Part model, mm, in its own coordinate system. A direction names the side the tool comes from. Round coordinates to 2 decimals unless told otherwise and drop trailing zeros. Order: outer loops, then holes, each group sorted by start corner. A loop starts at its lowest first (then second) coordinate and runs counter-clockwise, first axis right, second up. Notation, with made-up numbers: (1.25, -31) -> (51.25, -31) arc R24 ccw to (51.25, -12) -> close; hole circle Ø10 at (17, 19.25). An arc over 180 degrees is marked (long way). Answer as a JSON object with one key per item and string values. Group by question number.
```python
from build123d import *

# Parameters (mm, degrees)
SKETCH2_R           = 7.5
BOSS_EXTRUDE2_DEPTH = 80
SKETCH5_W           = 16
SKETCH5_H           = 60
CUT_EXTRUDE5_DEPTH  = 5
CUT_EXTRUDE6_DEPTH  = 28
CUT_EXTRUDE7_DEPTH  = 28
SKETCH8_R           = 2
CUT_EXTRUDE8_DEPTH  = 5


with BuildPart() as part:
    # Sketch2 → Boss-Extrude2 (new body)
    with BuildSketch(Plane.XY):
        Polygon((8, 0), (15, 0), (23.160384018, -17.5), (40, -17.5), (40, 17.5), (0, 17.5), (-40, 17.5), (-40, -17.5), (-23.160384018, -17.5), (-15, 0), (-8, 0), (-8, -5), (8, -5), align=None)
        with Locations((-27.5, 0)):
            Circle(SKETCH2_R, mode=Mode.SUBTRACT)
        with Locations((27.5, 0)):
            Circle(SKETCH2_R, mode=Mode.SUBTRACT)
        Polygon((-3, 0), (-3, -2.5), (3, -2.5), (3, 0), (3, 2.5), (-3, 2.5), align=None, mode=Mode.SUBTRACT)
    extrude(amount=-BOSS_EXTRUDE2_DEPTH)

    # Sketch5 → Cut-Extrude5 (cut)
    with BuildSketch(Plane(origin=(0, -5, 0), x_dir=(-1, 0, 0), z_dir=(0, -1, 0))):
        with Locations((0, 40)):
            Rectangle(SKETCH5_W, SKETCH5_H)
    extrude(amount=-CUT_EXTRUDE5_DEPTH, mode=Mode.SUBTRACT)

    # Sketch6 → Cut-Extrude6 (cut)
    with BuildSketch(Plane.XY):
        Polygon((-40, 12.5), (-40, -17.5), (-23.160384018, -17.5), (-15, 0), (-15, 12.5), align=None)
        Polygon((40, 12.5), (40, -17.5), (23.160384018, -17.5), (15, 0), (15, 12.5), align=None)
    extrude(amount=-CUT_EXTRUDE6_DEPTH, mode=Mode.SUBTRACT)

    # Sketch7 → Cut-Extrude7 (cut)
    with BuildSketch(Plane(origin=(0, 0, -80), x_dir=(-1, 0, 0), z_dir=(0, 0, -1))):
        Polygon((-40, 12.5), (-40, -17.5), (-23.160384018, -17.5), (-15, 0), (-15, 12.5), align=None)
        Polygon((40, 12.5), (40, -17.5), (23.160384018, -17.5), (15, 0), (15, 12.5), align=None)
    extrude(amount=-CUT_EXTRUDE7_DEPTH, mode=Mode.SUBTRACT)

    # Sketch8 → Cut-Extrude8 (cut)
    with BuildSketch(Plane(origin=(0, 17.5, 0), x_dir=(1, 0, 0), z_dir=(0, 1, 0))):
        with Locations(Location((27.5, 14, 0), (0, 0, 270))):
            Circle(SKETCH8_R)
        with Locations(Location((-27.5, 14, 0), (0, 0, 270))):
            Circle(SKETCH8_R)
        with Locations(Location((-27.5, 65.697240355, 0), (0, 0, 270))):
            Circle(SKETCH8_R)
        with Locations(Location((27.5, 65.697240355, 0), (0, 0, 270))):
            Circle(SKETCH8_R)
    extrude(amount=-CUT_EXTRUDE8_DEPTH, mode=Mode.SUBTRACT)


solid = part.part
```
Q1. Band-saw the part on C-C (y = 9). List the corners of the cut face in (x, z).
Q2. Band-saw the part on B-B (z = -50). List the corners of the cut face in (x, y).
Q3. Band-saw the part on A-A (x = -27.5). List the corners of the cut face in (y, z), plus the area to 3 significant figures.
Q4. Drop flat-ended pins along their axis: pin 1 Ø17 at (x, y) = (-27.5, 0) entering from -Z; pin 2 Ø5.5 at (y, z) = (-2, -6) entering from -X; pin 3 Ø2 at (y, z) = (-2.5, -70) entering from +X; pin 4 Ø9 at (x, y) = (27.5, 0) entering from -Z. Give the stop position or say it passes through.
Q5. Which spindle directions (+Z, -Z, +X, -X, +Y, -Y) get a long thin tool onto all of the face, cutting with end or side? Do faces 4 (the flat face through (-33, -6, -28)), 5 (the flat face through (-3, 1, -39)), 6 (the flat face through (8, -3, -5)), 7 (the flat face through (40, 4, -39)), 8 (the flat face through (15, 6, -14)). Say none if no direction does.
Q6. Band-saw the part on D-D (x = 34). List the corners of the cut face in (y, z).
Q7. Two-plate mould, pull along X, no slides. Class faces 1 (the flat face through (-19.137, -8.872, -39.832)), 2 (the flat face through (8, -3, -75)), 3 (the flat face through (31, -17.5, -40)): +X half, -X half, draft (parallel to the pull), parting line (faces both ways), or undercut.
Q8. Wall check: line 1 (X direction, y = 16, z = -14); line 2 (Z direction, x = 27, y = 15); line 3 (X direction, y = 1, z = -43). Give the ranges that are in metal, low to high. Write a range as [from, to].
Completed:
{
 "1": {"outline": "(-40, -52) -> (-15, -52) -> (-15, -80) -> (15, -80) -> (15, -52) -> (40, -52) -> (40, -28) -> (15, -28) -> (15, 0) -> (-15, 0) -> (-15, -28) -> (-40, -28) -> close"},
 "2": {"outline": "(-40, -17.5) -> (-23.16, -17.5) -> (-15, 0) -> (-3, 0) -> (-3, 2.5) -> (3, 2.5) -> (3, 0) -> (15, 0) -> (23.16, -17.5) -> (40, -17.5) -> (40, 17.5) -> (-40, 17.5) -> close; hole circle Ø15 at (-27.5, 0); hole circle Ø15 at (27.5, 0)"},
 "3": {"outline": "(-17.5, -52) -> (-7.5, -52) -> (-7.5, -28) -> (-17.5, -28) -> close; (7.5, -52) -> (12.5, -52) -> (12.5, -63.7) -> (17.5, -63.7) -> (17.5, -16) -> (12.5, -16) -> (12.5, -28) -> (7.5, -28) -> close; (12.5, -80) -> (17.5, -80) -> (17.5, -67.7) -> (12.5, -67.7) -> close; (12.5, -12) -> (17.5, -12) -> (17.5, 0) -> (12.5, 0) -> close", "area": "720 mm2"},
 "4": {"pin 1": "z = -52", "pin 2": "x = -15", "pin 3": "x = 8", "pin 4": "through"},
 "5": {"face 4": "+Z, -X, -Y", "face 5": "+Z, -Z", "face 6": "+Z, -Z, +X, -Y", "face 7": "+Z, -Z, +X, +Y, -Y", "face 8": "+Z, +X, -Y"},
 "6": {"outline": "(-17.5, -52) -> (-3.74, -52) -> (-3.74, -28) -> (-17.5, -28) -> close; (3.74, -52) -> (12.5, -52) -> (12.5, -80) -> (17.5, -80) -> (17.5, 0) -> (12.5, 0) -> (12.5, -28) -> (3.74, -28) -> close"},
 "7": {"face 1": "undercut", "face 2": "+X half", "face 3": "draft"},
 "8": {"line 1": "[-40, -29.5], [-25.5, 25.5], [29.5, 40]", "line 2": "[-80, -67.63], [-63.76, -15.94], [-12.06, 0]", "line 3": "[-40, -34.93], [-20.07, -3], [3, 20.07], [34.93, 40]"}
}
